The model under review builds one solid part; all positions refer to its coordinate system, in mm. A direction names the side the tool comes from. Round coordinates to 2 decimals unless told otherwise and drop trailing zeros. Write each loop counter-clockwise with the first axis right and the second up, starting at its lowest first coordinate (ties: lowest second). Pieces come first, ordered by that corner, then holes. Notation, with made-up numbers: (82, 63) - (106, 63) arc R31 ccw to (106, 88) - close; hole circle Ø9 at (40, 44.5). An arc over 180 degrees is marked (long way). Return JSON: item names as keys, results as strings.
from build123d import *

# Parameters (mm, degrees)
F0_W      = 45
F0_H      = 45
F1_DEPTH  = 5
F2_R      = 20
F3_DEPTH  = 9
F4_R      = 2
F5_DEPTH  = 25
F6_R      = 4
F7_DEPTH  = 25
F8_R      = 15.35
F9_DEPTH  = 25
F10_R     = 45.141628
F10_R_2   = 27.5
F11_DEPTH = 25


with BuildPart() as f1:
    # F0 (on Top) → F1 (new body)
    with BuildSketch(Plane.XY):
        Rectangle(F0_W, F0_H)
    extrude(amount=F1_DEPTH)

    # F2 (on face) → F3 (join)
    with BuildSketch(Plane.XY.offset(5)):
        Circle(F2_R)
    extrude(amount=F3_DEPTH)

    # F4 (on face) → F5 (cut)
    with BuildSketch(Plane(origin=(0, 0, 0), x_dir=(1, 0, 0), z_dir=(0, 0, -1))):
        with Locations((-15.5, 15.5)):
            Circle(F4_R)
        with Locations((-15.5, -15.5)):
            Circle(F4_R)
        with Locations((15.5, 15.5)):
            Circle(F4_R)
        with Locations((15.5, -15.5)):
            Circle(F4_R)
    extrude(amount=-F5_DEPTH, mode=Mode.SUBTRACT)

    # F6 (on face) → F7 (cut)
    with BuildSketch(Plane.XY.offset(5)):
        with Locations((15.5, -15.5)):
            Circle(F6_R)
        with Locations((-15.5, -15.5)):
            Circle(F6_R)
        with Locations((15.5, 15.5)):
            Circle(F6_R)
        with Locations((-15.5, 15.5)):
            Circle(F6_R)
    extrude(amount=F7_DEPTH, mode=Mode.SUBTRACT)

    # F8 (on face) → F9 (cut)
    with BuildSketch(Plane.XY.offset(14)):
        Circle(F8_R)
    extrude(amount=-F9_DEPTH, mode=Mode.SUBTRACT)

    # F10 (on face) → F11 (cut)
    with BuildSketch(Plane(origin=(0, 0, 0), x_dir=(1, 0, 0), z_dir=(0, 0, -1))):
        Circle(F10_R)
        Circle(F10_R_2, mode=Mode.SUBTRACT)
    extrude(amount=-F11_DEPTH, mode=Mode.SUBTRACT)


solid = f1.part
(1) Wall thickness on line 1 (X direction, y = 15.5, z = 3.85); line 2 (Y direction, x = 0, z = 9.5): over which ranges is each line inside the solid? List them lowest first.
Filled in:
{"line 1": "x = -22.5 to -17.5, -13.5 to 13.5, 17.5 to 22.5", "line 2": "y = -20 to -15.35, 15.35 to 20"}
(2) Mouldability with a two-part tool opening along Y and no side actions: class faces 4 (the cylindrical face through (19.4, 19.49, 2.46)), 5 (the cylindrical face through (19.49, -19.4, 2.46)), 6 (the cylindrical face through (12.711, -12.633, 9.437)) as released by +Y, released by -Y, zero draft, split by the parting line, or undercut.
Filled in:
{"face 4": "released by +Y", "face 5": "released by -Y", "face 6": "undercut"}
(3) Add section C-C (z = 8.5). Write out the cut boundary in (x, y), plus the area to 3 significant figures.
Filled in:
{"outline": "(-16.31, -11.58) arc R4 cw to (-11.58, -16.31) arc R20 ccw to (11.58, -16.31) arc R4 cw to (16.31, -11.58) arc R20 ccw to (16.31, 11.58) arc R4 cw to (11.58, 16.31) arc R20 ccw to (-11.58, 16.31) arc R4 cw to (-16.31, 11.58) arc R20 ccw to start; hole circle Ø30.7 at (0, 0)", "area": "478 mm2"}
(4) For faces 1 (the cylindrical face through (-20, 0, 9)), 2 (the cylindrical face through (0, 20, 9)), 3 (the cylindrical face through (-12.633, -12.711, 9.437)), list the 3-axis set-ups (+Z, -Z, +X, -X, +Y, -Y) from which the entire face can be reached by the end or side of a thin tool; tool diameter is ignored.
Filled in:
{"face 1": "+Z, -X", "face 2": "+Z, +Y", "face 3": "+Z"}
(5) Clearance check with flat-ended pins moving along their axes: pin 1 Ø6.5 at (x, y) = (-15.5, 15.5) entering from +Z; pin 2 Ø8 at (y, z) = (3.5, 12.5) entering from -X. State where each tip first meets the part, or that it passes through.
Filled in:
{"pin 1": "stops at z = 5", "pin 2": "stops at x = -20"}
(6) Add section A-A (x = 0). Write out the cut boundary in (y, z).
Filled in:
{"outline": "(-22.5, 0) - (-15.35, 0) - (-15.35, 14) - (-20, 14) - (-20, 5) - (-22.5, 5) - close; (15.35, 0) - (22.5, 0) - (22.5, 5) - (20, 5) - (20, 14) - (15.35, 14) - close"}
